Build history of the part. All positions in model axes, mm. A direction names the side the tool comes from. Round coordinates to 2 decimals unless told otherwise and drop trailing zeros. Write each loop counter-clockwise with the first axis right and the second up, starting at its lowest first coordinate (ties: lowest second). Pieces come first, ordered by that corner, then holes.
Item 1: Drop a flat-ended pin along its axis: pin 1 Ø8 at (x, y) = (13, -236) entering from +Z. Give the stop position or say it passes through.
Item 2: Band-saw the part on C-C, the plane x = 45. Write the cut outline in (y, z), then the cut area to 3 significant figures.
Item 3: 3-axis set-ups, long thin cutter, end or side, ignore diameter. For faces 1 (the flat face through (-4, 7, 0)), 2 (the flat face through (-280, -251, 331)): which of +Z, -Z, +X, -X, +Y, -Y reach the whole face in a straight line?
Item 4: Band-saw the part on B-B, the plane y = 208. Write the cut outline in (x, z).
Item 5: Wall check: probe 1 along X at (y, z) = (328, 126); probe 2 along Y at (x, z) = (230, 356); probe 3 along Z at (x, y) = (51.5, 154.5). Give the ranges that are in metal, low to high.
Item 6: Band-saw the part on A-A, the plane z = 555. Write the cut outline in (x, y), then the cut area to 4 significant figures.
```python
from build123d import *

# Parameters (mm, degrees)
SKETCH1_W           = 600
SKETCH1_H           = 1000
BOSS_EXTRUDE1_DEPTH = 650
SHELL1_T            = -20
BOSS_EXTRUDE2_REACH = 875.212
SKETCH2_W           = 5
SKETCH2_H           = 5


with BuildPart() as part:
    # Sketch1 → Boss-Extrude1 (new body)
    with BuildSketch(Plane.XY):
        Rectangle(SKETCH1_W, SKETCH1_H)
    extrude(amount=BOSS_EXTRUDE1_DEPTH)

    # Shell1
    shell1_openings = [part.faces().sort_by_distance(p)[0] for p in [
        (0, 0, 650),
    ]]
    offset(amount=SHELL1_T, openings=shell1_openings, kind=Kind.INTERSECTION)

    # Sketch2 → Boss-Extrude2 (add, up to next)
    with BuildSketch(Plane.XY.offset(650), mode=Mode.PRIVATE) as boss_extrude2_sk1:
        with Locations((-277.5, -12.5)):
            Rectangle(SKETCH2_W, SKETCH2_H)
    boss_extrude2_tool1 = extrude(boss_extrude2_sk1.sketch, amount=-BOSS_EXTRUDE2_REACH, mode=Mode.PRIVATE) - part.part
    # Sketch2 → Boss-Extrude2 (add, up to next)
    with BuildSketch(Plane.XY.offset(650), mode=Mode.PRIVATE) as boss_extrude2_sk2:
        with Locations((277.5, -12.5)):
            Rectangle(SKETCH2_W, SKETCH2_H)
    boss_extrude2_tool2 = extrude(boss_extrude2_sk2.sketch, amount=-BOSS_EXTRUDE2_REACH, mode=Mode.PRIVATE) - part.part
    add(boss_extrude2_tool1.solids().sort_by_distance((-277.5, -12.5, 650))[0])
    add(boss_extrude2_tool2.solids().sort_by_distance((277.5, -12.5, 650))[0])


solid = part.part
```
Results:
1. pin 1: stops at z = 20
2. outline: (-500, 0) - (500, 0) - (500, 650) - (480, 650) - (480, 20) - (-480, 20) - (-480, 650) - (-500, 650) - close
2. area: 45,200 mm2
3. face 1: -Z, +X, -X, +Y, -Y
3. face 2: +Z
4. outline: (-300, 0) - (300, 0) - (300, 650) - (280, 650) - (280, 20) - (-280, 20) - (-280, 650) - (-300, 650) - close
5. probe 1: x = -300 to -280, 280 to 300
5. probe 2: y = -500 to -480, 480 to 500
5. probe 3: z = 0 to 20
6. outline: (-300, -500) - (300, -500) - (300, 500) - (-300, 500) - close; hole (-280, -480) - (280, -480) - (280, -15) - (275, -15) - (275, -10) - (280, -10) - (280, 480) - (-280, 480) - (-280, -10) - (-275, -10) - (-275, -15) - (-280, -15) - close
6. area: 62,450 mm2
